Geometry: final body of the model. Coordinates: model frame, mm. Face numbers are marked on the shaded views. A direction names the side the tool comes from. Give positions to 0.01 mm unless a question says otherwise; leave off trailing zeros. Write each loop counter-clockwise with the first axis right and the second up, starting at its lowest first coordinate (ties: lowest second). Pieces come first, ordered by that corner, then holes.
Q1. Line query: line 1 (Z direction, x = 9, y = 25); line 2 (X direction, y = 25.65, z = -2.28); line 3 (X direction, y = 28, z = 2.5). Output: solid intervals per line, ascending.
Q2. Reachability of the marked faces 4, 5 and 6 from +Z, -Z, +X, -X, +Y, -Y: full face, straight path, thin tool, end or side. Return the list, or none.
Q3. Mould query, pull axis X, two halves, no side actions, for the marked faces 1, 2 and 3. Classes: +X half, -X half, draft (parallel to the pull), parting line (faces both ways), or undercut.
Q4. Section D-D (z = 1.5). Return the cut outline in (x, y), plus the area to 3 significant figures.
Q5. Section C-C (x = 33). Return the cut outline in (y, z).
Q6. Section A-A (y = 13). Return the cut outline in (x, z), plus the area to 3 significant figures.
Q7. Section B-B (z = -12.38). Return the cut outline in (x, y), plus the area to 3 significant figures.
Q8. Pin query (flat end, axial travel): pin 1 Ø2.5 at (x, z) = (56.8, -12.38) entering from -Y; pin 2 Ø16 at (x, y) = (5.5, 18.5) entering from +Z; pin 3 Ø14.5 at (x, z) = (60, 0) entering from +Y; pin 4 Ø8 at (x, z) = (50, -2) entering from -Y. Return the tip coordinate at first contact, or that it passes through.
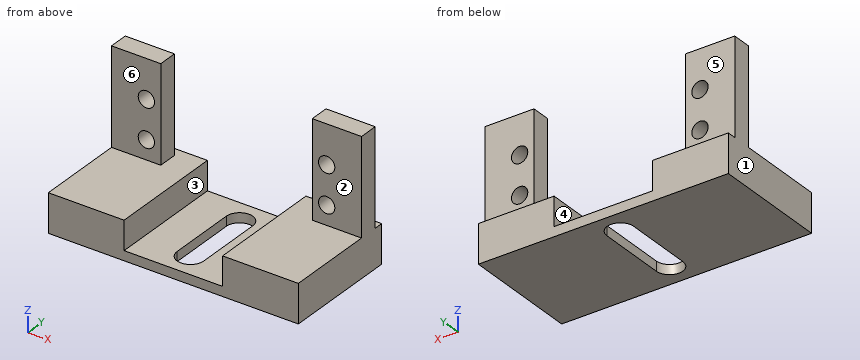
from build123d import *

# Parameters (mm, degrees)
SKETCH1_W           = 66
SKETCH1_H           = 27.619999878
BOSS_EXTRUDE1_DEPTH = 2.54
BOSS_EXTRUDE2_DEPTH = 26
SKETCH3_W           = 13
SKETCH3_H           = 5.08
BOSS_EXTRUDE3_DEPTH = 25.4
CUT_EXTRUDE1_REACH  = 78.124
CUT_EXTRUDE3_REACH  = 79.029
SKETCH5_R           = 2.15
BOSS_EXTRUDE4_DEPTH = 2.4
CUT_EXTRUDE4_REACH  = 82.023


with BuildPart() as part:
    # Sketch1 → Boss-Extrude1 (new body)
    with BuildSketch(Plane(origin=(0, 0, 0), x_dir=(1, 0, 0), z_dir=(0, 1, 0))):
        with Locations((33, 13.809999939)):
            Rectangle(SKETCH1_W, SKETCH1_H)
    extrude(amount=BOSS_EXTRUDE1_DEPTH)

    # Sketch2 → Boss-Extrude2 (add)
    with BuildSketch(Plane(origin=(0, 2.54, 0), x_dir=(1, 0, 0), z_dir=(0, 1, 0))):
        Polygon((0, 27.619999878), (66, 27.619999878), (66, 17.459999878), (46, 17.459999878), (46, 25.079999878), (20, 25.079999878), (20, 17.459999878), (0, 17.459999878), align=None)
    extrude(amount=BOSS_EXTRUDE2_DEPTH)

    # Sketch3 → Boss-Extrude3 (add)
    with BuildSketch(Plane.XY.offset(-17.459999878)):
        with Locations((6.5, 26)):
            Rectangle(SKETCH3_W, SKETCH3_H)
        with Locations((59.5, 26)):
            Rectangle(SKETCH3_W, SKETCH3_H)
    extrude(amount=BOSS_EXTRUDE3_DEPTH)

    # Sketch4 → Cut-Extrude1 (cut, up to next)
    with BuildSketch(Plane(origin=(0, 2.54, 0), x_dir=(1, 0, 0), z_dir=(0, 1, 0)), mode=Mode.PRIVATE) as cut_extrude1_sk1:
        Polygon((46, 17.459999878), (66, 17.459999878), (66, 0), (0, 0), (0, 17.459999878), (20, 17.459999878), (20, 25.079999878), (46, 25.079999878), align=None)
    cut_extrude1_tool1 = extrude(cut_extrude1_sk1.sketch, amount=-CUT_EXTRUDE1_REACH, mode=Mode.PRIVATE) & part.part
    add(cut_extrude1_tool1.solids().sort_by_distance((33, 2.54, -10.569661))[0], mode=Mode.SUBTRACT)

    # Sketch5 → Cut-Extrude3 (cut, up to next)
    with BuildSketch(Plane(origin=(0, 28.54, 0), x_dir=(1, 0, 0), z_dir=(0, 1, 0)), mode=Mode.PRIVATE) as cut_extrude3_sk1:
        with Locations(Location((56.8, 12.379999878, 0), (0, 0, 270))):
            Circle(SKETCH5_R)
    cut_extrude3_tool1 = extrude(cut_extrude3_sk1.sketch, amount=-CUT_EXTRUDE3_REACH, mode=Mode.PRIVATE) & part.part
    # Sketch5 → Cut-Extrude3 (cut, up to next)
    with BuildSketch(Plane(origin=(0, 28.54, 0), x_dir=(1, 0, 0), z_dir=(0, 1, 0)), mode=Mode.PRIVATE) as cut_extrude3_sk2:
        with Locations(Location((56.8, 2.279999878, 0), (0, 0, 270))):
            Circle(SKETCH5_R)
    cut_extrude3_tool2 = extrude(cut_extrude3_sk2.sketch, amount=-CUT_EXTRUDE3_REACH, mode=Mode.PRIVATE) & part.part
    cut_extrude3_1 = cut_extrude3_tool1.solids().sort_by_distance((56.8, 28.54, -12.38))[0]
    add(cut_extrude3_1, mode=Mode.SUBTRACT)
    cut_extrude3_2 = cut_extrude3_tool2.solids().sort_by_distance((56.8, 28.54, -2.28))[0]
    add(cut_extrude3_2, mode=Mode.SUBTRACT)
    cut_extrude3 = cut_extrude3_1 + cut_extrude3_2  # Cut-Extrude3 as one shape, for the pattern or mirror that repeats it

    # Mirror1: Cut-Extrude3 across plane
    add(cut_extrude3.mirror(Plane.ZY.offset(-33)), mode=Mode.SUBTRACT)

    # Sketch6 → Boss-Extrude4 (add)
    with BuildSketch(Plane(origin=(0, 28.54, 0), x_dir=(1, 0, 0), z_dir=(0, 1, 0))):
        Polygon((0, 27.619999878), (66, 27.619999878), (66, 17.459999878), (46, 17.459999878), (46, 25.079999878), (20, 25.079999878), (20, 17.459999878), (0, 17.459999878), align=None)
    extrude(amount=BOSS_EXTRUDE4_DEPTH)

    # Sketch7 → Cut-Extrude4 (cut, up to next)
    with BuildSketch(Plane.XY.offset(-25.079999878), mode=Mode.PRIVATE) as cut_extrude4_sk1:
        with BuildLine():
            Line((36.5, 24.59), (36.5, 6.35))
            ThreePointArc((36.5, 6.35), (33, 2.85), (29.5, 6.35))
            Line((29.5, 6.35), (29.5, 24.59))
            ThreePointArc((29.5, 24.59), (33, 28.09), (36.5, 24.59))
        make_face()
    cut_extrude4_tool1 = extrude(cut_extrude4_sk1.sketch, amount=-CUT_EXTRUDE4_REACH, mode=Mode.PRIVATE) & part.part
    add(cut_extrude4_tool1.solids().sort_by_distance((33, 15.47, -25.08))[0], mode=Mode.SUBTRACT)


solid = part.part
Computed:
1. line 1: z = -27.62 to -14.52, -10.24 to -4.42, -0.14 to 7.94
1. line 2: x = 0 to 7.05, 11.35 to 13, 53 to 54.65, 58.95 to 66
1. line 3: x = 0 to 13, 53 to 66
2. face 4: +Z, +Y, -Y
2. face 5: +Z, +X, -X, +Y
2. face 6: +Z, +X, -X, -Y
3. face 1: -X half
3. face 2: draft
3. face 3: undercut
4. outline: (0, 23.46) - (13, 23.46) - (13, 28.54) - (0, 28.54) - close; (53, 23.46) - (66, 23.46) - (66, 28.54) - (53, 28.54) - close
4. area: 132 mm2
5. outline: (0, -27.62) - (2.85, -27.62) - (2.85, -25.08) - (0, -25.08) - close; (28.09, -27.62) - (30.94, -27.62) - (30.94, -25.08) - (28.09, -25.08) - close
6. outline: (0, -27.62) - (29.5, -27.62) - (29.5, -25.08) - (20, -25.08) - (20, -17.46) - (0, -17.46) - close; (36.5, -27.62) - (66, -27.62) - (66, -17.46) - (46, -17.46) - (46, -25.08) - (36.5, -25.08) - close
6. area: 455 mm2
7. outline: (0, 23.46) - (7.05, 23.46) - (7.05, 28.54) - (0, 28.54) - close; (11.35, 23.46) - (13, 23.46) - (13, 28.54) - (11.35, 28.54) - close; (53, 23.46) - (54.65, 23.46) - (54.65, 28.54) - (53, 28.54) - close; (58.95, 23.46) - (66, 23.46) - (66, 28.54) - (58.95, 28.54) - close
7. area: 88.4 mm2
8. pin 1: passes through
8. pin 2: stops at z = 7.94
8. pin 3: stops at y = 28.54
8. pin 4: stops at y = 23.46
